Autodesk Inventor part; units mm, degrees
ref_plane "Arbeitsebene2" through (-4.46, 32.72, -4) normal (0, 0, 1) x (1, 0, 0)
ref_plane "YZ Plane" through (0, 0, 0) normal (1, 0, 0) x (0, 1, 0)
ref_plane "XZ Plane" through (0, 0, 0) normal (0, 1, 0) x (-1, 0, 0)
ref_plane "Arbeitsebene1" through (0, 0, 0) normal (0, 0, 1) x (1, 0, 0)
sketch "Skizze1" plane through (0, 0, 0) normal (0, 0, 1) x (1, 0, 0)
  circle A0 centre (-64.84, -24.91) radius 1.5
  circle A1 centre (85.34, -22.83) radius 1
  circle A2 centre (85.34, -43.41) radius 1
  circle A3 centre (-64.84, 35.59) radius 1.5
  circle A4 centre (-11.66, -50.59) radius 1.5
  circle A5 centre (85.34, 37.77) radius 1
  circle A6 centre (54.34, -50.59) radius 1.5
  circle A7 centre (85.34, 58.59) radius 1
  line L0 (-89.84, 67.09) -> (89.84, 67.09)
  line L1 (-89.84, -67.09) -> (-89.84, 67.09)
  line L2 (89.84, -67.09) -> (-89.84, -67.09)
  line L3 (89.84, 67.09) -> (89.84, -67.09)
  arc A8 (-32.14, 53.27) -> (-37.14, 48.27) centre (-32.14, 48.27) ccw
  line L4 (73.22, 53.27) -> (-32.14, 53.27)
  arc A9 (78.22, 48.27) -> (73.22, 53.27) centre (73.22, 48.27) ccw
  line L5 (78.22, -36.73) -> (78.22, 48.27)
  arc A10 (73.22, -41.73) -> (78.22, -36.73) centre (73.22, -36.73) ccw
  line L6 (-32.14, -41.73) -> (73.22, -41.73)
  arc A11 (-37.14, -36.73) -> (-32.14, -41.73) centre (-32.14, -36.73) ccw
  line L7 (-37.14, 48.27) -> (-37.14, -36.73)
  circle A12 centre (37.4417, 38.67) radius 1.75
  circle A13 centre (24.9417, 38.67) radius 1.75
  circle A14 centre (12.4417, 38.67) radius 1.75
  circle A15 centre (-0.0583, 38.67) radius 1.75
  line L8 (-4.46, 32.72) -> (-4.46, 44.82) construction
  line L9 (-4.46, 32.72) -> (45.54, 32.72)
  line L10 (45.54, 32.72) -> (45.54, 44.82) construction
  line L11 (-4.46, 44.82) -> (45.54, 44.82)
  circle A16 centre (36, 49.77) radius 1
  circle A17 centre (10.54, 48.77) radius 1.25
  line L12 (55.54, 52.32) -> (-14.46, 52.32)
  line L13 (-14.46, 52.32) -> (-14.46, 25.22)
  line L14 (-14.46, 25.22) -> (55.54, 25.22)
  line L15 (55.54, 25.22) -> (55.54, 52.32)
  circle A18 centre (20.54, 38.77) radius 1.4
  circle A19 centre (33.04, 38.77) radius 1.4
  circle A20 centre (45.54, 38.77) radius 1.4
  circle A21 centre (8.04, 38.77) radius 1.4
  circle A22 centre (20.54, 38.77) radius 1.4
  circle A23 centre (33.04, 38.77) radius 1.4
  circle A24 centre (-4.46, 38.77) radius 1.4
  circle A25 centre (8.04, 38.77) radius 1.4
  circle A26 centre (20.54, 38.77) radius 1.4
  point P0 (0, 0)
  dimension "d0" = 10
  dimension "d1" = 10
  dimension "d2" = 7.5
  dimension "d3" = 7.5
  dimension "d4" = 2.8
  dimension "d7" = 12.5
  dimension "d10" = 12.5
ref_plane "Arbeitsebene2" through (-4.46, 32.72, -4) normal (0, 0, 1) x (1, 0, 0)
extrude "Extrusion1" add sketch "Skizze1" against normal blind 6 contours A12 | A13 | A14 | A15 | L15 L14 L13 L12
sketch "Skizze2" plane through (55.54, 25.22, -6) normal (0, 0, -1) x (-1, 0, 0)
  circle A0 centre (19.54, 24.55) radius 1
  circle A1 centre (55.54, 24.55) radius 1
  point P0 (55.54, -25.22)
hole "Bohrung1" at (0, 49.77, -6) at (36, 49.77, -6) direction (0, 0, 1) diameter 2 end through all counterbore diameter 4.5 counterbore depth 2
sketch "Skizze3" plane through (55.54, 25.22, 0) normal (1, 0, 0) x (0, 0, -1)
  line L0 (0, 27.1) -> (6, 27.1)
  line L1 (4, 27.1) -> (4, 0)
  line L2 (0, 0) -> (6, 0)
  line L3 (4, 0) -> (36, 0)
  line L4 (36, 0) -> (36, 27.1)
  line L5 (36, 27.1) -> (4, 27.1)
  line L6 (4, 27.1) -> (4, 0)
  circle A0 centre (31.0266, 13.55) radius 3.005 construction
  circle A1 centre (31.0266, 13.55) radius 2.8511 construction
  circle A2 centre (31.0266, 13.55) radius 2.6
  point P0 (0, -25.22)
  dimension "d22" = 32
  dimension "d44" = 5.2
extrude "Extrusion2" add sketch "Skizze3" against normal blind 7
chamfer "Fase1" distance 5 angle 45 2 edges at (52.04, 52.32, -36) (52.04, 25.22, -36)
sketch "Skizze4" plane through (-14.46, 52.32, -36) normal (0, 0, -1) x (1, 0, 0)
  circle A0 centre (66.1385, 17.6805) radius 1.4
  line L0 (69.238, 10.6988) -> (61.364, 10.6988)
  line L1 (69.238, 16.4011) -> (61.364, 16.4011)
  circle A1 centre (66.1385, 9.4552) radius 1.4
  point P0 (14.46, 52.32)
  dimension "d30" = 2.8
  dimension "d41" = 2.8
ref_plane "Arbeitsebene3" through (0, 0, -12.82) normal (0, 0, -1) x (-1, 0, 0)
extrude "Extrusion4" cut sketch "Skizze4" against normal blind 15
properties part number "30_XYTabel_Aliexpress_cellSTORM_xmount"
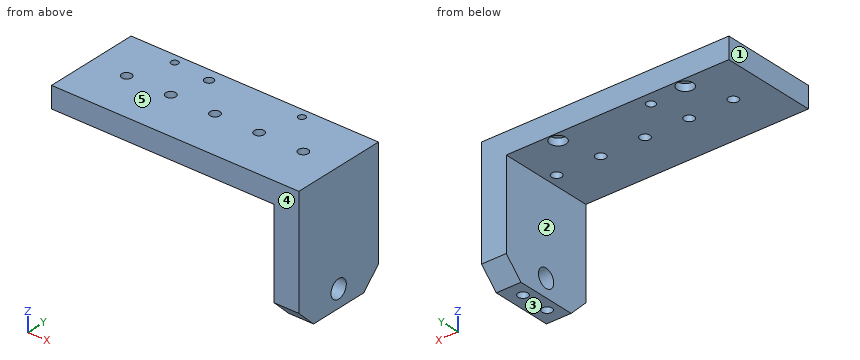
Read the model definition and answer for the solid it produces. Units are mm, in the model's axes. Face numbers are marked on the shaded views. A direction names the side the tool comes from. Round coordinates to 2 decimals unless told otherwise and drop trailing zeros. Write each loop counter-clockwise with the first axis right and the second up, starting at its lowest first coordinate (ties: lowest second). Pieces come first, ordered by that corner, then holes.
1. Given pin 1 Ø1.6 at (x, y) = (36, 49.77) entering from +Z; pin 2 Ø3.5 at (x, y) = (8.04, 38.77) entering from -Z; pin 3 Ø3.5 at (x, y) = (36, 49.77) entering from -Z; pin 4 Ø8 at (y, z) = (43.5, -20.5) entering from -X, each flat-ended and moving along its own axis, determine where each tip first touches the part or whether it passes through.
2. Which of the six approach directions +Z, -Z, +X, -X, +Y, -Y give full straight-line access (tool end or side, diameter ignored) to the marked faces 1 and 2?
3. The part is cut by section D-D, the plane z = -12.5. Determine the outline of the cut face in (x, y), then the cut area to 3 significant figures.
4. Determine the mould class of the marked faces 3, 4 and 5 for opening direction Z: pulls with the +Z half, pulls with the -Z half, needs draft (parallel to the pull), parting line crosses it, or undercut.
5. The part is cut by section B-B, the plane z = -3. State how many separate pieces and enclosed holes the cut face has, then the cut area to 3 significant figures.
6. Straight lines are drawn through the part: L1, parallel to Y at x = 51, z = -25; L2, parallel to Y at x = 20.54, z = -4.3; L3, parallel to X at y = 31, z = -10. For each, find the intervals that lie inside material, in ascending order.
7. The part is cut by section C-C, the plane x = 0. Determine the outline of the cut face in (y, z).
8. The part is cut by section A-A, the plane x = 45.54. Determine the outline of the cut face in (y, z).
Values:
1. pin 1: passes through
1. pin 2: stops at z = -6
1. pin 3: stops at z = -4
1. pin 4: stops at x = 48.54
2. face 1: +Z, -Z, -X, +Y, -Y
2. face 2: -Z, -X, +Y, -Y
3. outline: (48.54, 25.22) - (55.54, 25.22) - (55.54, 52.32) - (48.54, 52.32) - close
3. area: 190 mm2
4. face 3: pulls with the -Z half
4. face 4: needs draft
4. face 5: pulls with the +Z half
5. separate pieces: 1
5. enclosed holes: 8
5. area: 1,860 mm2
6. L1: y = 25.22 to 33.41, 35.86 to 41.64, 44.09 to 52.32
6. L2: y = 25.22 to 37.37, 40.17 to 52.32
6. L3: x = 48.54 to 55.54
7. outline: (25.22, -6) - (47.52, -6) - (47.52, -4) - (48.77, -4) - (48.77, 0) - (25.22, 0) - close; (50.77, -4) - (52.02, -4) - (52.02, -6) - (52.32, -6) - (52.32, 0) - (50.77, 0) - close
8. outline: (25.22, -6) - (37.37, -6) - (37.37, 0) - (25.22, 0) - close; (40.17, -6) - (52.32, -6) - (52.32, 0) - (40.17, 0) - close
